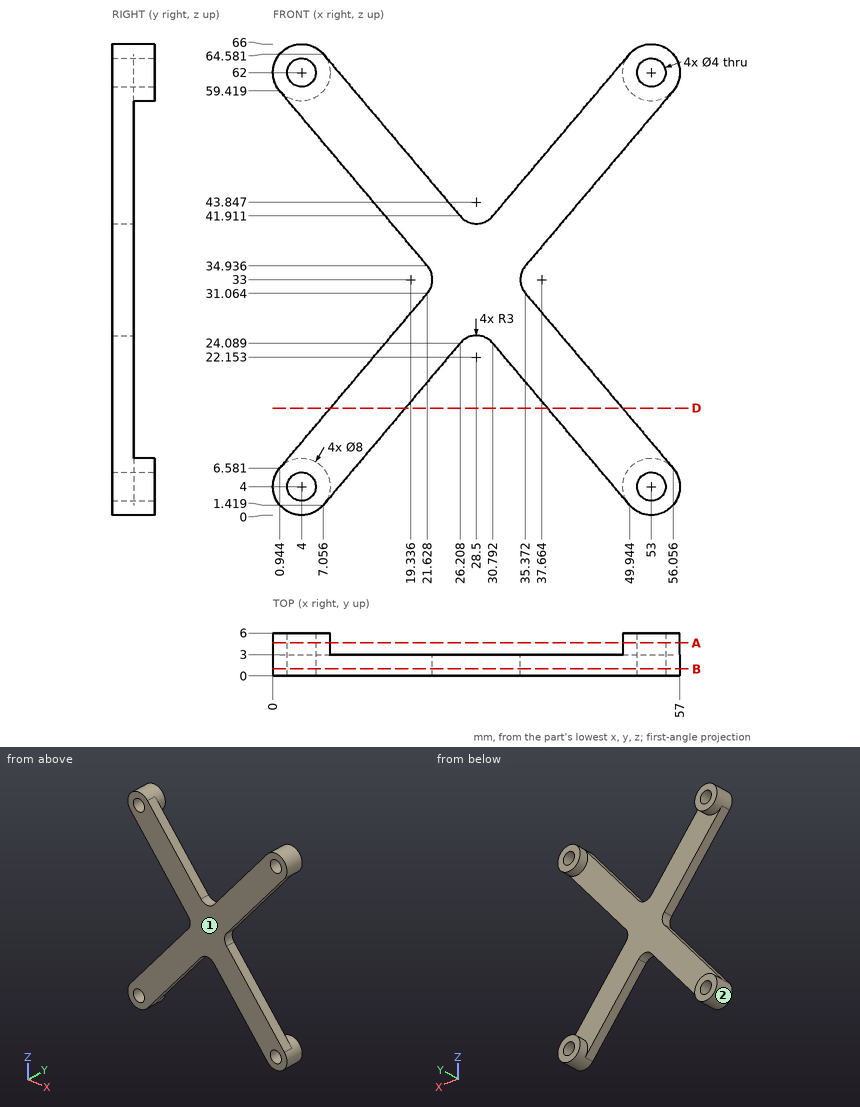
Source: three-view drawing plus pictorial views. Frame: mm from the lowest corner of the part. Give positions to 0.01 mm unless a question says otherwise; leave off trailing zeros. Write each loop counter-clockwise with the first axis right and the second up, starting at its lowest first coordinate (ties: lowest second). Pieces come first, ordered by that corner, then holes. Notation, with made-up numbers: M 25,58.25 L 58,58.25 A31 ccw 58,83.25 Z; hole C -22,-40 d10. An arc over 180 degrees is marked long. Use one line per item in the form item = value.
1. Cut plane B-B on y = 1. Return loops of the section in (x, z) (1 decimal).
Outcome:
outline = M 0.9,6.6 A4 ccw 7.1,1.4 L 26.2,24.1 A3 cw 30.8,24.1 L 49.9,1.4 A4 ccw 56.1,6.6 L 35.4,31.1 A3 cw 35.4,34.9 L 56.1,59.4 A4 ccw 49.9,64.6 L 30.8,41.9 A3 cw 26.2,41.9 L 7.1,64.6 A4 ccw 0.9,59.4 L 21.6,34.9 A3 cw 21.6,31.1 Z; hole C 4,4 d4; hole C 4,62 d4; hole C 53,4 d4; hole C 53,62 d4
2. Mould query, pull axis Z, two halves, no side actions, for the marked faces 1 and 2. Classes: released by +Z, released by -Z, zero draft, split by the parting line, or undercut.
Outcome:
face_1 = zero draft
face_2 = undercut
3. Cut plane A-A on y = 4.65. Return loops of the section in (x, z), and give its area (3 significant figures).
Outcome:
outline = C 4,4 d8; C 4,62 d8; C 53,4 d8; C 53,62 d8; hole C 4,4 d4; hole C 4,62 d4; hole C 53,4 d4; hole C 53,62 d4
area = 151 mm²
4. First-contact query: P1, Ø3, axis at x = 42.5, z = 23, coming from the +Y side. Flat tip, straight axial feed; report the tip coordinate or a pass-through.
Outcome:
P1 = 3
5. Ray query, L1, parallel to Z at x = 52.5, y = 2.5 (1 decimal); L2, parallel to Z at x = 51.5, y = 3.85 (1 decimal); L3, parallel to Y at x = 47, z = 7. Return the intervals inside material, ascending.
Outcome:
L1 = 0 to 2.1, 5.9 to 10.8, 55.2 to 60.1, 63.9 to 66
L2 = 0.3 to 2.7, 5.3 to 7.7, 58.3 to 60.7, 63.3 to 65.7
L3 = 0 to 3
6. Cut plane D-D on z = 15. Return loops of the section in (x, y).
Outcome:
outline = M 8.06,0 L 18.53,0 L 18.53,3 L 8.06,3 Z; M 38.47,0 L 48.94,0 L 48.94,3 L 38.47,3 Z
